Autodesk Inventor part; units mm, degrees
ref_plane "YZ Plane" through (0, 0, 0) normal (1, 0, 0) x (0, 1, 0)
ref_plane "XZ Plane" through (0, 0, 0) normal (0, 1, 0) x (-1, 0, 0)
ref_plane "XY Plane" through (0, 0, 0) normal (0, 0, 1) x (1, 0, 0)
sketch "Sketch1" plane through (0, 0, 0) normal (0, 0, 1) x (1, 0, 0)
  line L0 (0, 0) -> (20, 0)
  line L1 (20, 0) -> (20, 37)
  line L2 (20, 37) -> (0, 37)
  line L3 (0, 37) -> (0, 0)
  dimension "d0" = 20
  dimension "d1" = 37
extrude "Extrusion1" add sketch "Sketch1" along normal blind 5
sketch "Sketch2" plane through (0, 0, 5) normal (0, 0, 1) x (1, 0, 0)
  line L0 (20, 0) -> (0, 0)
  line L1 (20, 37) -> (20, 0)
  point P0 (10, 26)
  dimension "d4" = 26
  dimension "d5" = 10
hole "Hole1" at (10, 26, 5) direction (0, 0, -1) diameter 12 depth 5 tip angle 118
fillet "Fillet1" radius 10 2 edges at (20, 37, 2.5) (0, 37, 2.5)
sketch "Sketch3" plane through (0, 0, 5) normal (0, 0, 1) x (1, 0, 0)
  line L0 (0, 0) -> (0, 27)
  line L1 (20, 0) -> (0, 0)
  point P0 (10, 10)
  dimension "d14" = 10
  dimension "d15" = 10
hole "Hole2" at (10, 10, 5) direction (0, 0, -1) diameter 4.917 depth 6 tip angle 118
chamfer "Chamfer1" distance 0.5 angle 45 2 edges at (10, 12.4585, 5) (10, 12.4585, 0)
properties part number "SUPORTE DO EIXO TRASEIRO(51)" material "Carbon Steel"
Build history of the part. All positions in model axes, mm. Round coordinates to 2 decimals unless told otherwise and drop trailing zeros. Write each loop counter-clockwise with the first axis right and the second up, starting at its lowest first coordinate (ties: lowest second). Pieces come first, ordered by that corner, then holes.
1) Band-saw the part on C-C, the plane y = 26. List the corners of the cut face in (x, z), and give its area (3 significant figures).
2) Band-saw the part on A-A, the plane y = 10. List the corners of the cut face in (x, z), and give its area (3 significant figures).
3) Band-saw the part on B-B, the plane z = 1.45. Give the number of separate pieces and of enclosed holes in the cut face, and give its area (3 significant figures).
4) Band-saw the part on D-D, the plane x = 17.5. List the corners of the cut face in (y, z).
5) Pin check, flat tip, straight feed: pin 1 (6.5 mm diameter, centred on x = 10, y = 10, fed in from -Z). Stop position of the tip, or through.
6) Mould opens along X. For faces 1 (the flat face through (0, 14, 2)), 2 (the flat face through (20, 13, 2)), 3 (the cylindrical face through (5.94, 30.42, 2.46)), 4 (the cylindrical face through (8.338, 11.812, 2.472)) say: +X half, -X half, draft (parallel to the pull), parting line (faces both ways), or undercut.
7) Drill centre lines: probe 1 along Y at (x, z) = (10, 2.6); probe 2 along X at (y, z) = (10, 2.85); probe 3 along X at (y, z) = (26, 4). Where is each one in solid material? Low to high.
Ans:
1. outline: (0, 0) - (4, 0) - (4, 5) - (0, 5) - close; (16, 0) - (20, 0) - (20, 5) - (16, 5) - close
1. area: 40.0 mm2
2. outline: (0, 0) - (7.04, 0) - (7.54, 0.5) - (7.54, 4.5) - (7.04, 5) - (0, 5) - close; (12.46, 0.5) - (12.96, 0) - (20, 0) - (20, 5) - (12.96, 5) - (12.46, 4.5) - close
2. area: 74.9 mm2
3. separate pieces: 1
3. enclosed holes: 2
3. area: 565 mm2
4. outline: (0, 0) - (33.61, 0) - (33.61, 5) - (0, 5) - close
5. pin 1: stops at z = 0
6. face 1: -X half
6. face 2: +X half
6. face 3: undercut
6. face 4: undercut
7. probe 1: y = 0 to 7.54, 12.46 to 20, 32 to 37
7. probe 2: x = 0 to 7.54, 12.46 to 20
7. probe 3: x = 0 to 4, 16 to 20
